Geometry check sheet. Reference: the model listing, model coordinates, mm. Round coordinates to 2 decimals unless told otherwise and drop trailing zeros. Write each loop counter-clockwise with the first axis right and the second up, starting at its lowest first coordinate (ties: lowest second). Pieces come first, ordered by that corner, then holes. Notation, with made-up numbers: (32, -23) - (47, -23) arc R20 cw to (47, -8) - close; hole circle Ø7 at (9, -30.5). An arc over 180 degrees is marked (long way). Return JSON: item names as keys, results as strings.
Autodesk Inventor part; units mm, degrees
ref_plane "YZ Plane" through (0, 0, 0) normal (1, 0, 0) x (0, 1, 0)
ref_plane "XZ Plane" through (0, 0, 0) normal (0, 1, 0) x (-1, 0, 0)
ref_plane "XY Plane" through (0, 0, 0) normal (0, 0, 1) x (1, 0, 0)
sketch "Sketch1" plane through (0, 0, 0) normal (0, 1, 0) x (-1, 0, 0)
  line L0 (-75, 10) -> (75, 10)
  line L1 (75, 10) -> (75, -10)
  line L2 (75, -10) -> (-75, -10)
  line L3 (-75, -10) -> (-75, 10)
  line L4 (-75, 10) -> (75, -10) construction
  line L5 (75, 10) -> (-75, -10) construction
  point P0 (0, 0)
  dimension "Length" = 150
  dimension "Width" = 20
extrude "Extrusion1" add sketch "Sketch1" along normal mid plane 10
sketch "Sketch4" plane through (0, 5, 0) normal (0, 1, 0) x (1, 0, 0)
  point P0 (0, 0)
  point P1 (-60, 0)
  point P2 (60, 0)
  dimension "d16" = 120
  dimension "d17" = 60
hole "Hole2" at (-60, 5, 0) at (60, 5, 0) direction (0, -1, 0) diameter 9 end through all
fillet "Fillet1" radius 5 4 edges at (75, 0, 10) (75, 0, -10) (-75, 0, 10) (-75, 0, -10)
chamfer "Chamfer2" distance 0.5 angle 45 8 edges at (0, 5, 10) (73.5355, 5, 8.5355) (75, 5, 0) (73.5355, 5, -8.5355) (0, 5, -10) (-73.5355, 5, -8.5355) (-75, 5, 0) (-73.5355, 5, 8.5355)
properties part number "Lower Arm Brass Plate - 3" material "Brass, Soft Yellow"
(1) Release check for a two-part mould opening along X. For faces 1 (the face through (75, 0, 0)), 2 (the face through (1, -5, 0)), 3 (the face through (63.99, -0.07, 2.08)) record: pulls with the +X half, pulls with the -X half, needs draft (parallel to the pull), parting line crosses it, or undercut.
Response values:
{"face 1": "pulls with the +X half", "face 2": "needs draft", "face 3": "undercut"}
(2) Section check C-C, the plane y = -0.25. Enter the section's corners in (x, z).
Response values:
{"outline": "(-75, -5) arc R5 ccw to (-70, -10) - (70, -10) arc R5 ccw to (75, -5) - (75, 5) arc R5 ccw to (70, 10) - (-70, 10) arc R5 ccw to (-75, 5) - close; hole circle Ø9 at (-60, 0); hole circle Ø9 at (60, 0)"}
(3) Gauge pin test, flat end, axial feed: pin 1 (1.5 mm diameter, centred on y = -1, z = 7.5, fed in from -X). Record the tip position at first contact, or that the pin passes through.
Response values:
{"pin 1": "stops at x = -74.68"}
(4) Section check B-B, the plane z = 0. Enter the section's corners in (x, y), plus the area to 3 significant figures.
Response values:
{"outline": "(-75, -5) - (-64.5, -5) - (-64.5, 5) - (-74.5, 5) - (-75, 4.5) - close; (-55.5, -5) - (55.5, -5) - (55.5, 5) - (-55.5, 5) - close; (64.5, -5) - (75, -5) - (75, 4.5) - (74.5, 5) - (64.5, 5) - close", "area": "1,320 mm^2"}
(5) Section check A-A, the plane x = -60. Enter the section's corners in (y, z).
Response values:
{"outline": "(-5, -10) - (4.5, -10) - (5, -9.5) - (5, -4.5) - (-5, -4.5) - close; (-5, 4.5) - (5, 4.5) - (5, 9.5) - (4.5, 10) - (-5, 10) - close"}
(6) Material ranges on line 1 along X through (y, z) = (-1, 0); line 2 along X through (y, z) = (1.5, 3.25); line 3 along Z through (x, y) = (-60, 0.75), recorded low to high. Write a range as [from, to].
Response values:
{"line 1": "x = [-75, -64.5], [-55.5, 55.5], [64.5, 75]", "line 2": "x = [-75, -63.11], [-56.89, 56.89], [63.11, 75]", "line 3": "z = [-10, -4.5], [4.5, 10]"}
